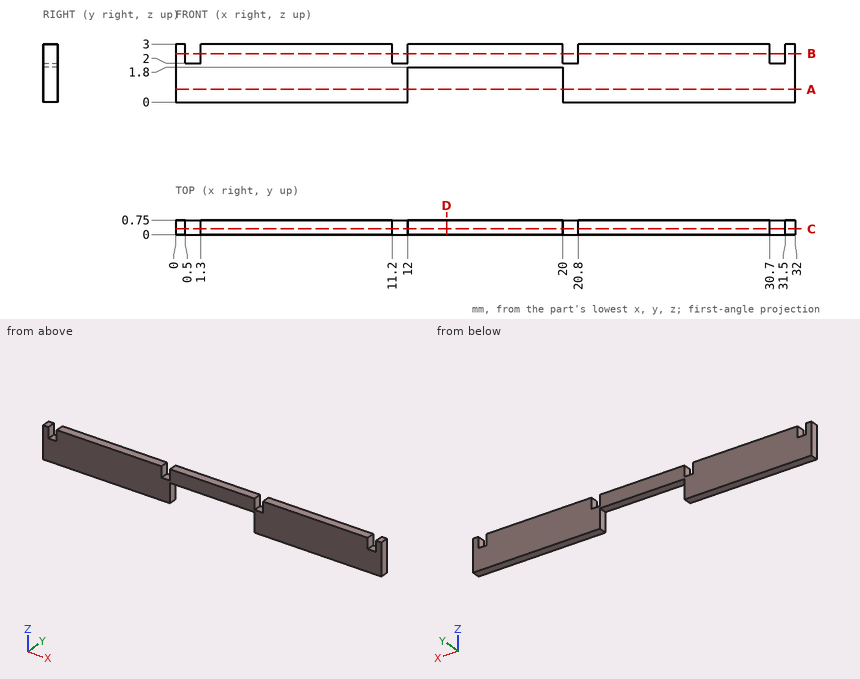
Answer from the drawing. Dimensions are ordinates in mm from the lowest x, y and z of the part. Coordinates: 2 decimals unless noted, no trailing zeros. Order: outer loops, then holes, each group sorted by start corner. A loop starts at its lowest first (then second) coordinate and runs counter-clockwise, first axis right, second up. Notation, with made-up numbers: (35, 45.5) - (45, 45.5) arc R14 cw to (45, 52.5) - close; hole circle Ø8 at (64.25, 3). An arc over 180 degrees is marked (long way). Answer as a JSON object with one key per item and string values. Group by question number.
Item 1: Consider probe 1 along X at (y, z) = (0.45, 2.85); probe 2 along X at (y, z) = (0.4, 0.8); probe 3 along Z at (x, y) = (19.5, 0.1). Determine where each line is inside the solid, lowest interval first. Write a range as from..to.
Item 2: Section D-D (x = 14) is taken. Give the vertices of the cut face in (y, z), plus the area to 3 significant figures.
Item 3: Section C-C (y = 0.3) is taken. Give the vertices of the cut face in (x, z), plus the area to 3 significant figures.
Item 4: Section A-A (z = 0.65) is taken. Give the vertices of the cut face in (x, y), plus the area to 3 significant figures.
Item 5: Section B-B (z = 2.5) is taken. Give the vertices of the cut face in (x, y), plus the area to 3 significant figures.
Results are:
{
 "1": {"probe 1": "x = 0..0.5, 1.3..11.2, 12..20, 20.8..30.7, 31.5..32", "probe 2": "x = 0..12, 20..32", "probe 3": "z = 1.8..3"},
 "2": {"outline": "(0, 1.8) - (0.75, 1.8) - (0.75, 3) - (0, 3) - close", "area": "0.900 mm^2"},
 "3": {"outline": "(0, 0) - (12, 0) - (12, 1.8) - (20, 1.8) - (20, 0) - (32, 0) - (32, 3) - (31.5, 3) - (31.5, 2) - (30.7, 2) - (30.7, 3) - (20.8, 3) - (20.8, 2) - (20, 2) - (20, 3) - (12, 3) - (12, 2) - (11.2, 2) - (11.2, 3) - (1.3, 3) - (1.3, 2) - (0.5, 2) - (0.5, 3) - (0, 3) - close", "area": "78.4 mm^2"},
 "4": {"outline": "(0, 0) - (12, 0) - (12, 0.75) - (0, 0.75) - close; (20, 0) - (32, 0) - (32, 0.75) - (20, 0.75) - close", "area": "18.0 mm^2"},
 "5": {"outline": "(0, 0) - (0.5, 0) - (0.5, 0.75) - (0, 0.75) - close; (1.3, 0) - (11.2, 0) - (11.2, 0.75) - (1.3, 0.75) - close; (12, 0) - (20, 0) - (20, 0.75) - (12, 0.75) - close; (20.8, 0) - (30.7, 0) - (30.7, 0.75) - (20.8, 0.75) - close; (31.5, 0) - (32, 0) - (32, 0.75) - (31.5, 0.75) - close", "area": "21.6 mm^2"}
}
